Geometry check sheet. Reference: the model listing, model coordinates, mm. A direction names the side the tool comes from. Round coordinates to 2 decimals unless told otherwise and drop trailing zeros. Loops run counter-clockwise (first coordinate to the right, second up) from the corner with the lowest first, then second, coordinate; pieces in that order, holes last. Notation, with made-up numbers: M 39.5,42 L 50.5,42 A18 cw 50.5,55 Z; hole C 17,17 d3. An arc over 180 degrees is marked long. Use one line per item in the form item = value. Start each with the question number.
1. Go/stop test with flat-tipped pins: pin 1 (1.1 mm diameter, centred on x = 0.5, z = 0.5, fed in from -Y); pin 2 (2 mm diameter, centred on y = 4.5, z = 0.5, fed in from +X); pin 3 (5 mm diameter, centred on x = -2, y = 7.5, fed in from +Z); pin 4 (1.5 mm diameter, centred on x = 2, y = 11, fed in from -Z). Record where each tip stops, or that it passes through.
2. Material ranges on line 1 (Y direction, x = -0.25, z = -0.6); line 2 (Z direction, x = 3.25, y = 12.75); line 3 (Z direction, x = 5.25, y = 9.25), recorded low to high.
3. Cross-section at A-A (y = 3.5). Record the boundary of the cut face in (x, z).
4. Set-up check for faces 1 (the cylindrical face through (-0.488, 1.972, -0.108)), 2 (the flat face through (0, 19, 0)): record each of +Z, -Z, +X, -X, +Y, -Y from which the full face is reachable in a straight line by a thin tool's end or side.
```python
from build123d import *

# Parameters (mm, degrees)
SKETCH1_R           = 0.5
BOSS_EXTRUDE1_DEPTH = 4


with BuildPart() as part:
    # Sketch1 → Boss-Extrude1 (new body)
    with BuildSketch(Plane(origin=(0, 0, 0), x_dir=(1, 0, 0), z_dir=(0, 1, 0))):
        with Locations(Location((0, 0, 0), (0, 0, 270))):
            Circle(SKETCH1_R)
    extrude(amount=BOSS_EXTRUDE1_DEPTH)

    # Loft1: read off the stored shape, not the designer's step
    # Loft1: loft between two sections, ruled curve by curve
    loft1_from = [
        Edge.make_bspline([(3.982375398, 4, 1.293952205), (3.778342255, 4, 1.041167834), (3.35743147, 4, 0.747073774), (2.774835702, 4, 0.481725971), (2.388912903, 4, 0.307417574), (1.943119665, 4, 0.114072033), (1.491029323, 4, -0.05934005), (0.918025904, 4, -0.291830044), (0.582544384, 4, -0.445572937), (0.091107981, 4, -0.648252812), (-0.215529223, 4, -0.758866155), (-0.712050383, 4, -0.892823244), (-1.051235123, 4, -0.958457066), (-1.583065933, 4, -1.00758396), (-1.864928757, 4, -0.950412973), (-2.177884928, 4, -0.708144109), (-2.327212912, 4, -0.335223441), (-2.097184928, 4, -0.059033354), (-2, 4, 0)], [0, 0, 0, 0, 0.126695771, 0.206989258, 0.254842699, 0.296675286, 0.40244821, 0.449001509, 0.545040751, 0.551021467, 0.66150331, 0.674317156, 0.759992592, 0.804387527, 0.871243058, 0.872553131, 0.965343615, 1, 1, 1, 1], 3),
        Edge.make_bspline([(-2, 4, 0), (-1.898005082, 4, 0.025463399), (-1.598012325, 4, 0.098239141), (-1.082098728, 4, 0.213990908), (-0.305813383, 4, 0.373809131), (0.518693331, 4, 0.530338625), (1.38750976, 4, 0.695180106), (2.080405352, 4, 0.833106398), (2.710695257, 4, 0.969417149), (3.313517993, 4, 1.111722031), (3.735710336, 4, 1.223446834), (3.974512186, 4, 1.291699256), (3.982375398, 4, 1.293952205)], [0, 0, 0, 0, 0.051489964, 0.151232112, 0.259137033, 0.439966352, 0.562511328, 0.692507299, 0.786234451, 0.878581378, 0.996001399, 1, 1, 1, 1], 3),
    ]
    loft1_to = [
        Edge.make_bspline([(7.945912088, 19, 2.558825735), (7.999326678, 19, 2.379766219), (6.586617231, 19, 1.514362157), (5.583308433, 19, 0.929295889), (4.970659737, 19, 0.599281473), (4.193046499, 19, 0.202001465), (3.341628587, 19, -0.206134907), (2.283698675, 19, -0.693976723), (1.657446394, 19, -0.966026664), (0.745558302, 19, -1.333617961), (0.178585745, 19, -1.542245386), (-0.764999991, 19, -1.784056092), (-1.423521481, 19, -1.897535409), (-2.337702573, 19, -1.96274037), (-2.858978808, 19, -1.956236967), (-3.606715655, 19, -1.786802244), (-4.20333017, 19, -1.473764254), (-4.400691171, 19, -0.863287732), (-4.422732973, 19, -0.693782032)], [0, 0, 0, 0, 0.126695771, 0.206989258, 0.254842699, 0.296675286, 0.40244821, 0.449001509, 0.545040751, 0.551021467, 0.66150331, 0.674317156, 0.759992592, 0.804387527, 0.871243058, 0.872553131, 0.965343615, 1, 1, 1, 1], 3),
        Edge.make_bspline([(-4.422732973, 19, -0.693782032), (-4.454247575, 19, -0.451428682), (-4.356921525, 19, 0.281406104), (-3.124219807, 19, 0.833691628), (-1.42226489, 19, 0.797143302), (0.430553453, 19, 0.848586825), (2.360686602, 19, 1.14455408), (3.788192091, 19, 1.717620789), (5.223115534, 19, 2.036792165), (6.310537615, 19, 2.445358722), (7.869311301, 19, 2.719580004), (7.944289787, 19, 2.564264106), (7.945912088, 19, 2.558825735)], [0, 0, 0, 0, 0.051489964, 0.151232112, 0.259137033, 0.439966352, 0.562511328, 0.692507299, 0.786234451, 0.878581378, 0.996001399, 1, 1, 1, 1], 3),
    ]
    loft1 = Solid(Shell([*[Face.make_surface_from_curves(loft1_from[k], loft1_to[k]) for k in range(2)], Face(Wire(loft1_from)), Face(Wire(loft1_to))]))
    add(loft1)


solid = part.part
```
Reported:
q1.pin_1 = 0
q1.pin_2 = 4.24
q1.pin_3 = 0.62
q1.pin_4 = -0.62
q2.line_1 = 4 to 19
q2.line_2 = 0.17 to 1.37
q2.line_3 = 1.58 to 1.73
q3.outline = C 0,0 d1
q4.face_1 = -Y
q4.face_2 = +Z, -Z, +X, -X, +Y
